from build123d import *

# Parameters (mm, degrees)
SKETCH1_R           = 12.2
BOSS_EXTRUDE1_DEPTH = 12.4
SKETCH2_R           = 1
BOSS_EXTRUDE2_DEPTH = 7
SKETCH3_R           = 3.2
BOSS_EXTRUDE3_DEPTH = 1
SKETCH4_W           = 4
SKETCH4_H           = 4
SKETCH4_R           = 0.75
BOSS_EXTRUDE4_DEPTH = 12.5
FILLET1_R           = 1


with BuildPart() as part:
    # Sketch1 → Boss-Extrude1 (new body)
    with BuildSketch(Plane.XY):
        Circle(SKETCH1_R)
    extrude(amount=BOSS_EXTRUDE1_DEPTH)

    # Sketch2 → Boss-Extrude2 (add)
    with BuildSketch(Plane.XY.offset(12.4)):
        Circle(SKETCH2_R)
    extrude(amount=BOSS_EXTRUDE2_DEPTH)

    # Sketch3 → Boss-Extrude3 (add)
    with BuildSketch(Plane.XY.offset(12.4)):
        Circle(SKETCH3_R)
    extrude(amount=BOSS_EXTRUDE3_DEPTH)

    # Sketch4 → Boss-Extrude4 (add)
    with BuildSketch(Plane(origin=(0, 0, 0), x_dir=(0, 0, -1), z_dir=(1, 0, 0))):
        with Locations((-2, 0)):
            Rectangle(SKETCH4_W, SKETCH4_H)
        with Locations((-3, 1)):
            Circle(SKETCH4_R, mode=Mode.SUBTRACT)
        with Locations((-3, -1)):
            Circle(SKETCH4_R, mode=Mode.SUBTRACT)
    extrude(amount=-BOSS_EXTRUDE4_DEPTH)

    # Fillet1
    fillet1_edges = [part.edges().sort_by_distance(p)[0] for p in [
        (-12.2, 0, 12.4),
    ]]
    fillet(fillet1_edges, radius=FILLET1_R)


solid = part.part
Can you work these out from the model? Positions are in its coordinate system, mm. A direction names the side the tool comes from. Coordinates: 2 decimals unless noted, no trailing zeros. Loops run counter-clockwise (first coordinate to the right, second up) from the corner with the lowest first, then second, coordinate; pieces in that order, holes last. Notation, with made-up numbers: M 86.25,-8 L 104.25,-8 A23 ccw 104.25,5 Z; hole C -16,60.5 d11. An arc over 180 degrees is marked long. Answer as CSV lines item,"result". Start each with the question number.
1. If I drill on probe 1 along Y at (x, z) = (-12.3, 3); probe 2 along Z at (x, y) = (-12.2, 1); probe 3 along X at (y, z) = (0.25, 5.25), over which ranges is the centre line in solid material (lowest first)? Write a range as [from, to].
2. Suppose I cut it at B-B, the plane z = 16.5. List the corners of the cut face in (x, y) for me, plus the area to 3 significant figures.
3. Thinking about a two-plate mould opening in Z: for faces 1 (the face through (-12.5, 0, 2)), 2 (the face through (0, 0, 19.4)), 3 (the face through (-12.331, 1.744, 3.098)), which applies, +Z half, -Z half, draft (parallel to the pull), parting line (faces both ways), or undercut?
4. For pin 1 Ø3 at (x, y) = (7, -1.5) entering from +Z; pin 2 Ø1.2 at (y, z) = (1, 3) entering from -X; pin 3 Ø6 at (y, z) = (6, 17) entering from -X; pin 4 Ø1 at (x, z) = (-7.5, 12.5) entering from -Y, each with a flat end and sliding along its axis, tell me the tip position at first contact or that it passes through.
5. Suppose I cut it at C-C, the plane z = 7. List the corners of the cut face in (x, y) for me.
6. For faces 4 (the face through (0, 0, 0)), 5 (the face through (-12.331, -1.732, 3.163)), 6 (the face through (1, 1, 13.4)), which set-ups out of +Z, -Z, +X, -X, +Y, -Y let a thin tool reach every point of the face, with its end or its side?
7. Suppose I cut it at A-A, the plane z = 3. List the corners of the cut face in (x, y) for me, plus the area to 3 significant figures.
Output:
1,probe 1,"y = [-2, -1.75], [-0.25, 0.25], [1.75, 2]"
1,probe 2,"z = [0, 2.25], [3.75, 4]"
1,probe 3,"x = [-12.2, 12.2]"
2,outline,"C 0,0 d2"
2,area,"3.14 mm^2"
3,face 1,"draft"
3,face 2,"+Z half"
3,face 3,"undercut"
4,pin 1,"stops at z = 12.4"
4,pin 2,"stops at x = -12.19"
4,pin 3,"passes through"
4,pin 4,"stops at y = -9.49"
5,outline,"C 0,0 d24.4"
6,face 4,"-Z, +X, -X, +Y, -Y"
6,face 5,"-X"
6,face 6,"+Z"
7,outline,"M -12.5,-2 L -12.03,-2 A12.2 ccw long -12.03,2 L -12.5,2 L -12.5,1.75 L -12.07,1.75 A12.2 ccw -12.2,0.25 L -12.5,0.25 L -12.5,-0.25 L -12.2,-0.25 A12.2 ccw -12.07,-1.75 L -12.5,-1.75 Z"
7,area,"468 mm^2"
